For this review, take the finished solid that the model builds, in its own axes (mm). Face numbers are marked on the shaded views. A direction names the side the tool comes from. Round coordinates to 2 decimals unless told otherwise and drop trailing zeros. Write each loop counter-clockwise with the first axis right and the second up, starting at its lowest first coordinate (ties: lowest second). Pieces come first, ordered by that corner, then holes. Notation, with made-up numbers: (-27.5, -10.75) - (21.5, -10.75) arc R19 ccw to (21.5, 15.25) - close; hole circle Ø10 at (-1, 25.5). An arc over 180 degrees is marked (long way). Answer in a Markdown table with one row per item. Add a question column.
from build123d import *

# Parameters (mm, degrees)
SKETCH1_W           = 11
SKETCH1_H           = 28
BOSS_EXTRUDE1_DEPTH = 10
SKETCH2_R           = 3
CUT_EXTRUDE1_DEPTH  = 5
SKETCH3_W           = 5
SKETCH3_H           = 5
CUT_EXTRUDE2_DEPTH  = 1
FILLET1_R           = 2
BOSS_EXTRUDE2_DEPTH = 10
BOSS_EXTRUDE3_DEPTH = 5
SKETCH6_W           = 9
SKETCH6_H           = 24
SKETCH6_W_2         = 5
SKETCH6_H_2         = 5
BOSS_EXTRUDE4_DEPTH = 4


with BuildPart() as part:
    # Sketch1 → Boss-Extrude1 (new body)
    with BuildSketch(Plane(origin=(0, 0, 0), x_dir=(1, 0, 0), z_dir=(0, 1, 0))):
        with Locations((5.5, 14)):
            Rectangle(SKETCH1_W, SKETCH1_H)
    extrude(amount=BOSS_EXTRUDE1_DEPTH)

    # Sketch2 → Cut-Extrude1 (cut)
    with BuildSketch(Plane.XZ):
        with Locations(Location((5.5, -6, 0), (0, 0, 270))):  # turned: the seam where the file's is
            Circle(SKETCH2_R)
        with Locations(Location((5.5, -22, 0), (0, 0, 90))):  # turned: the seam where the file's is
            Circle(SKETCH2_R)
    extrude(amount=-CUT_EXTRUDE1_DEPTH, mode=Mode.SUBTRACT)

    # Sketch3 → Cut-Extrude2 (cut)
    with BuildSketch(Plane(origin=(0, 10, 0), x_dir=(1, 0, 0), z_dir=(0, 1, 0))):
        with Locations((5.5, 8.8)):
            Rectangle(SKETCH3_W, SKETCH3_H)
        with Locations((5.5, 19.2)):
            Rectangle(SKETCH3_W, SKETCH3_H)
    extrude(amount=-CUT_EXTRUDE2_DEPTH, mode=Mode.SUBTRACT)

    # Fillet1
    fillet1_edges = [part.edges().sort_by_distance(p)[0] for p in [
        (0, 5, -28),
        (11, 5, -28),
        (11, 5, 0),
        (0, 5, 0),
    ]]
    fillet(fillet1_edges, radius=FILLET1_R)

    # Sketch4 → Boss-Extrude2 (add)
    with BuildSketch(Plane(origin=(0, 10, 0), x_dir=(1, 0, 0), z_dir=(0, 1, 0))):
        Polygon((-7, 10), (3, 10), (3, 11.3), (8, 11.3), (8, 10), (18, 10), (18, 18), (8, 18), (8, 16.7), (3, 16.7), (3, 18), (-7, 18), align=None)
    extrude(amount=-BOSS_EXTRUDE2_DEPTH)

    # Sketch5 → Boss-Extrude3 (add, symmetric)
    with BuildSketch(Plane(origin=(0, 0, -14), x_dir=(-1, 0, 0), z_dir=(0, 0, -1))):
        with BuildLine():
            Line((-18, 10), (-18, 14))
            Line((-18, 14), (-23.009639132, 14))
            ThreePointArc((-23.009639132, 14), (-23.034060421, 13.203534611), (-23.107232535, 12.410061639))
            ThreePointArc((-23.107232535, 12.410061639), (-24.247773279, 11.621237367), (-23.503399625, 10.451201135))
            ThreePointArc((-23.503399625, 10.451201135), (-23.712034257, 9.784680991), (-23.956162944, 9.130327344))
            ThreePointArc((-23.956162944, 9.130327344), (-25.254024229, 8.659499735), (-24.844635532, 7.340968944))
            ThreePointArc((-24.844635532, 7.340968944), (-25.19276603, 6.789226373), (-25.568138069, 6.255643632))
            ThreePointArc((-25.568138069, 6.255643632), (-27.002153814, 6.177218324), (-26.878916821, 4.74635693))
            ThreePointArc((-26.878916821, 4.74635693), (-27.400685234, 4.259059964), (-27.948418079, 3.801141479))
            ThreePointArc((-27.948418079, 3.801141479), (-29.288657634, 4.007780534), (-29.602553888, 2.688534194))
            ThreePointArc((-29.602553888, 2.688534194), (-30.295715938, 2.323053407), (-31.009639132, 2))
            Line((-31.009639132, 2), (-31.009639132, 0))
            Line((-31.009639132, 0), (-18, 0))
            Line((-18, 0), (-18, 10))
        make_face()
    boss_extrude3 = extrude(amount=BOSS_EXTRUDE3_DEPTH, both=True)

    # Mirror1: Boss-Extrude3 across plane
    add(boss_extrude3.mirror(Plane.ZY.offset(-5.5)))

    # Sketch6 → Boss-Extrude4 (add)
    with BuildSketch(Plane(origin=(0, 10, 0), x_dir=(1, 0, 0), z_dir=(0, 1, 0))):
        with Locations((5.5, 14)):
            Rectangle(SKETCH6_W, SKETCH6_H)
        with Locations((5.5, 19.2)):
            Rectangle(SKETCH6_W_2, SKETCH6_H_2, mode=Mode.SUBTRACT)
        with Locations((5.5, 8.8)):
            Rectangle(SKETCH6_W_2, SKETCH6_H_2, mode=Mode.SUBTRACT)
    extrude(amount=BOSS_EXTRUDE4_DEPTH)


solid = part.part
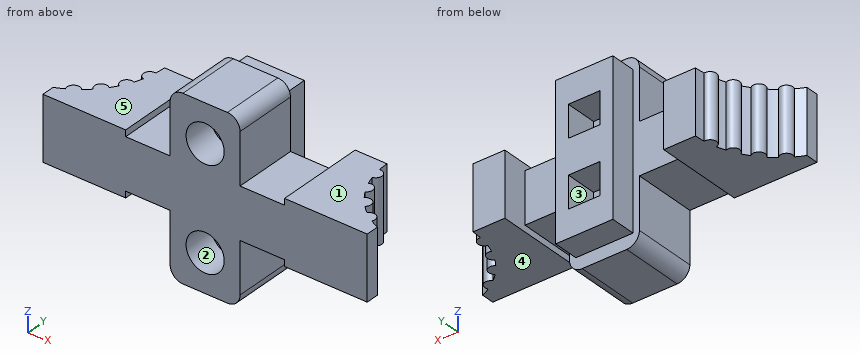
Q1. Add section D-D on z = -7.5. State the section outline as (x, y) points, then the cut area to 3 significant figures.
Q2. To check wall thickness, follow probe 1 along X at (y, z) = (11.5, -18); probe 2 along X at (y, z) = (12, -21); probe 3 along X at (y, z) = (2.25, -22). State the ranges of each line that lie inside material, in increasing order.
Q3. Add section A-A on x = 5.5. State the section outline as (y, z) points.
Q4. Tool access review of the marked faces 1, 2, 3, 4 and 5: name each direction out of +Z, -Z, +X, -X, +Y, -Y from which nothing blocks a thin tool from reaching the whole face with its end or side.
Q5. Insertion check: pin 1 Ø4 at (y, z) = (11.5, -12) entering from +X; pin 2 Ø4 at (y, z) = (6.5, -11.5) entering from +X; pin 3 Ø2 at (x, y) = (13, 4) entering from -Z. Each pin has a flat end and moves straight along its axis. Give the tip position at first contact, or say it passes through.
Q6. Add section C-C on y = 5.5. State the section outline as (x, z) points.
Answer sheet:
| question | item | result |
|---|---|---|
| 1 | outline | (0, 0) - (2.9, 0) - (2.9, 5) - (8.1, 5) - (8.1, 0) - (11, 0) - (11, 10) - (10, 10) - (10, 14) - (8, 14) - (8, 9) - (3, 9) - (3, 14) - (1, 14) - (1, 10) - (0, 10) - close |
| 1 | area | 95.0 mm² |
| 2 | probe 1 | x = -13.26 to -7, 1 to 3, 8 to 10, 18 to 24.26 |
| 2 | probe 2 | x = 1 to 3, 8 to 10 |
| 2 | probe 3 | x = 0 to 2.5, 8.5 to 11 |
| 3 | outline | (0, -28) - (10, -28) - (10, -26) - (14, -26) - (14, -21.7) - (9, -21.7) - (9, -16.7) - (14, -16.7) - (14, -11.3) - (9, -11.3) - (9, -6.3) - (14, -6.3) - (14, -2) - (10, -2) - (10, 0) - (0, 0) - (0, -3) - (5, -3) - (5, -9) - (0, -9) - (0, -19) - (5, -19) - (5, -25) - (0, -25) - close |
| 4 | face 1 | +Z, +X, +Y, -Y |
| 4 | face 2 | -Y |
| 4 | face 3 | +Y |
| 4 | face 4 | -Z, +X, +Y, -Y |
| 4 | face 5 | +Z, -X, +Y, -Y |
| 5 | pin 1 | stops at x = 24.27 |
| 5 | pin 2 | stops at x = 27.25 |
| 5 | pin 3 | stops at z = -18 |
| 6 | outline | (-16.25, -19) - (-7, -19) - (-7, -18) - (0, -18) - (0, -26) arc R2 ccw to (2, -28) - (9, -28) arc R2 ccw to (11, -26) - (11, -18) - (18, -18) - (18, -19) - (27.25, -19) - (27.25, -9) - (18, -9) - (18, -10) - (11, -10) - (11, -2) arc R2 ccw to (9, 0) - (2, 0) arc R2 ccw to (0, -2) - (0, -10) - (-7, -10) - (-7, -9) - (-16.25, -9) - close |
